Verification items for the finished model (mm, model axes). A direction names the side the tool comes from. Give positions to 0.01 mm unless a question says otherwise; leave off trailing zeros. Loops run counter-clockwise (first coordinate to the right, second up) from the corner with the lowest first, then second, coordinate; pieces in that order, holes last. Notation, with made-up numbers: M 13,-32.5 L 26,-32.5 A6 ccw 26,-24.5 Z; hole C 14.25,-33 d2. An arc over 180 degrees is marked long. Put each result on its own line as item: value. Start each with the question number.
Autodesk Inventor part; units mm, degrees
ref_plane "YZ Plane" through (0, 0, 0) normal (1, 0, 0) x (0, 1, 0)
ref_plane "XZ Plane" through (0, 0, 0) normal (0, 1, 0) x (-1, 0, 0)
ref_plane "XY Plane" through (0, 0, 0) normal (0, 0, 1) x (1, 0, 0)
sketch "Sketch1" plane through (0, 0, 0) normal (0, 0, 1) x (1, 0, 0)
  line L0 (-44.4426, 24.9959) -> (-36.4426, 24.9959)
  line L1 (-36.4426, 24.9959) -> (-36.4426, -13.0041)
  line L2 (-36.4426, -13.0041) -> (-44.4426, -13.0041)
  line L3 (-44.4426, -13.0041) -> (-44.4426, 24.9959)
  point P0 (0, 0)
  dimension "d0" = 38
  dimension "d2" = 8
extrude "Extrusion1" add sketch "Sketch1" along normal blind 3
sketch "Sketch2" plane through (0, 0, 3) normal (0, 0, 1) x (1, 0, 0)
  line L0 (-44.4426, 24.9959) -> (-44.4426, -13.0041) construction
  line L1 (-44.4426, -13.0041) -> (-36.4426, -13.0041)
  line L2 (-36.4426, -13.0041) -> (-36.4426, 24.9959)
  line L3 (-44.4426, 24.9959) -> (-36.4426, 24.9959)
  line L4 (-36.4426, 24.9959) -> (-36.4426, 15.2459)
  line L5 (-36.4426, 15.2459) -> (-44.4426, 15.2459)
  line L6 (-44.4426, 15.2459) -> (-44.4426, 24.9959)
  line L7 (-36.4426, -13.0041) -> (-44.4426, -13.0041)
  line L8 (-44.4426, -13.0041) -> (-44.4426, -3.2541)
  line L9 (-44.4426, -3.2541) -> (-36.4426, -3.2541)
  line L10 (-36.4426, -3.2541) -> (-36.4426, -13.0041)
  point P0 (0, 0)
  dimension "d5" = 9.75
  dimension "d7" = 9.75
extrude "Extrusion2" add sketch "Sketch2" along normal blind 6.5
sketch "Sketch3" plane through (0, 0, 9.5) normal (0, 0, 1) x (1, 0, 0)
  line L0 (-36.4426, -13.0041) -> (-36.4426, -3.2541)
  line L1 (-36.4426, -3.2541) -> (-44.4426, -3.2541)
  line L2 (-44.4426, -3.2541) -> (-44.4426, -13.0041)
  line L3 (-44.4426, -13.0041) -> (-36.4426, -13.0041)
  line L4 (-36.4426, 24.9959) -> (-44.4426, 15.2459) construction
  line L5 (-36.4426, -3.2541) -> (-44.4426, -13.0041) construction
  circle A0 centre (-40.4426, 20.1209) radius 1.65
  circle A1 centre (-40.4426, -8.1291) radius 1.65
  point P0 (0, 0)
  dimension "d10" = 3.3
extrude "Extrusion3" cut sketch "Sketch3" against normal through all contours A0 | A1
properties part number "Pump clamp MM0312"
Q1. Release check for a two-part mould opening along Y. For faces 3 (the face through (-40, 15.246, 6)), 4 (the face through (-40, -13.004, 5)), 5 (the face through (-42.3, 20.2, 9.5)) record: pulls with the +Y half, pulls with the -Y half, needs draft (parallel to the pull), parting line crosses it, or undercut.
Q2. Scan lines: L1, parallel to Y at x = -40.5, z = 6.5; L2, parallel to Y at x = -42.25, z = 8.25; L3, parallel to Z at x = -42, y = 7.5. Record each from-to range of solid material in increasing order.
Q3. Cross-section at A-A, the plane z = 3.5. Record the boundary of the cut face in (x, y).
Q4. Set-up check for faces 1 (the face through (-40, -3.254, 6)), 2 (the face through (-42.3, -8.1, 9.5)): record each of +Z, -Z, +X, -X, +Y, -Y from which the full face is reachable in a straight line by a thin tool's end or side.
Q5. Cross-section at D-D, the plane z = 2. Record the boundary of the cut face in (x, y).
Q6. Cross-section at C-C, the plane x = -38.25. Record the boundary of the cut face in (y, z).
Q7. Cross-section at B-B, the plane x = -40.75. Record the boundary of the cut face in (y, z).
Ans:
1. face 3: undercut
1. face 4: pulls with the -Y half
1. face 5: needs draft
2. L1: y = -13 to -9.78, -6.48 to -3.25, 15.25 to 18.47, 21.77 to 25
2. L2: y = -13 to -3.25, 15.25 to 25
2. L3: z = 0 to 3
3. outline: M -44.44,-13 L -36.44,-13 L -36.44,-3.25 L -44.44,-3.25 Z; M -44.44,15.25 L -36.44,15.25 L -36.44,25 L -44.44,25 Z; hole C -40.44,-8.13 d3.3; hole C -40.44,20.12 d3.3
4. face 1: +Z, +X, -X
4. face 2: +Z, +X, -X, +Y, -Y
5. outline: M -44.44,-13 L -36.44,-13 L -36.44,25 L -44.44,25 Z; hole C -40.44,-8.13 d3.3; hole C -40.44,20.12 d3.3
6. outline: M -13,0 L 25,0 L 25,9.5 L 15.25,9.5 L 15.25,3 L -3.25,3 L -3.25,9.5 L -13,9.5 Z
7. outline: M -13,0 L -9.75,0 L -9.75,9.5 L -13,9.5 Z; M -6.51,0 L 18.5,0 L 18.5,9.5 L 15.25,9.5 L 15.25,3 L -3.25,3 L -3.25,9.5 L -6.51,9.5 Z; M 21.74,0 L 25,0 L 25,9.5 L 21.74,9.5 Z
